from build123d import *

# Parameters (mm, degrees)
BOX011_W          = 6.2
BOX011_H          = 10
BOX011_DEPTH      = 2.4
BOX010_W          = 6.2
BOX010_H          = 10
BOX010_DEPTH      = 2.4
CYLINDER007_R     = 1.5
CYLINDER007_DEPTH = 60
CYLINDER006_R     = 4.5
CYLINDER006_DEPTH = 60


with BuildPart() as nut2:
    # Box011 → Box011 (new body)
    with BuildSketch(Plane(origin=(-3.1, -5, 51.6), x_dir=(1, 0, 0), z_dir=(0, 0, 1))):
        with Locations((3.1, 5)):
            Rectangle(BOX011_W, BOX011_H)
    extrude(amount=BOX011_DEPTH)


with BuildPart() as nut1:
    # Box010 → Box010 (new body)
    with BuildSketch(Plane(origin=(-3.1, -5, 6), x_dir=(1, 0, 0), z_dir=(0, 0, 1))):
        with Locations((3.1, 5)):
            Rectangle(BOX010_W, BOX010_H)
    extrude(amount=BOX010_DEPTH)


with BuildPart() as columnhole:
    # Cylinder007 → Cylinder007 (new body)
    with BuildSketch(Plane.XY):
        Circle(CYLINDER007_R)
    extrude(amount=CYLINDER007_DEPTH)


with BuildPart() as column:
    # Cylinder006 → Cylinder006 (new body)
    with BuildSketch(Plane.XY):
        Circle(CYLINDER006_R)
    extrude(amount=CYLINDER006_DEPTH)

    # Cut010: cut ColumnHole
    add(columnhole.part, mode=Mode.SUBTRACT)

    # Cut011: cut Nut1
    add(nut1.part, mode=Mode.SUBTRACT)

    # Cut012: cut Nut2
    add(nut2.part, mode=Mode.SUBTRACT)


solid = column.part
The listing builds one solid part. Answer for the finished solid, in the listing's coordinates (mm). A direction names the side the tool comes from. Round coordinates to 2 decimals unless told otherwise and drop trailing zeros. Loops run counter-clockwise (first coordinate to the right, second up) from the corner with the lowest first, then second, coordinate; pieces in that order, holes last. Notation, with made-up numbers: M 45.25,-34 L 73.25,-34 A32 cw 73.25,4 Z; hole C 13.25,86.5 d1. An arc over 180 degrees is marked long. Return JSON: item names as keys, results as strings.
Q1. Find the intervals of material crossed by line 1 along Z through (x, y) = (-2, 3); line 2 along Y through (x, z) = (0, 49); line 3 along X through (y, z) = (-0.75, 33), in increasing order. Write a range as from..to.
Results list:
{"line 1": "z = 0..6, 8.4..51.6, 54..60", "line 2": "y = -4.5..-1.5, 1.5..4.5", "line 3": "x = -4.44..-1.3, 1.3..4.44"}
Q2. Find section A-A, the plane x = 0. Determine the outline of the cut face in (y, z), plus the area to 3 significant figures.
Results list:
{"outline": "M -4.5,0 L -1.5,0 L -1.5,6 L -4.5,6 Z; M -4.5,8.4 L -1.5,8.4 L -1.5,51.6 L -4.5,51.6 Z; M -4.5,54 L -1.5,54 L -1.5,60 L -4.5,60 Z; M 1.5,0 L 4.5,0 L 4.5,6 L 1.5,6 Z; M 1.5,8.4 L 4.5,8.4 L 4.5,51.6 L 1.5,51.6 Z; M 1.5,54 L 4.5,54 L 4.5,60 L 1.5,60 Z", "area": "331 mm2"}
Q3. Find section B-B, the plane y = 0.5. Determine the outline of the cut face in (x, z).
Results list:
{"outline": "M -4.47,0 L -1.41,0 L -1.41,6 L -3.1,6 L -3.1,8.4 L -1.41,8.4 L -1.41,51.6 L -3.1,51.6 L -3.1,54 L -1.41,54 L -1.41,60 L -4.47,60 Z; M 1.41,0 L 4.47,0 L 4.47,60 L 1.41,60 L 1.41,54 L 3.1,54 L 3.1,51.6 L 1.41,51.6 L 1.41,8.4 L 3.1,8.4 L 3.1,6 L 1.41,6 Z"}
Q4. Find section C-C, the plane x = 2.5. Determine the outline of the cut face in (y, z).
Results list:
{"outline": "M -3.74,0 L 3.74,0 L 3.74,6 L -3.74,6 Z; M -3.74,8.4 L 3.74,8.4 L 3.74,51.6 L -3.74,51.6 Z; M -3.74,54 L 3.74,54 L 3.74,60 L -3.74,60 Z"}
Q5. Find section D-D, the plane z = 53. Determine the outline of the cut face in (x, y), plus the area to 3 significant figures.
Results list:
{"outline": "M -3.1,-3.26 L -3.1,3.26 A4.5 ccw Z; M 3.1,-3.26 A4.5 ccw 3.1,3.26 Z", "area": "12.6 mm2"}
Q6. The mould has two halves that part along X. Classify faces 3 (the face through (3.1, 0, 53)), 4 (the face through (-1.5, 0.07, 29.7)), 5 (the face through (0, -2, 0)), 6 (the face through (-0.59, 4.46, 29.58)): released by +X, released by -X, zero draft, split by the parting line, or undercut.
Results list:
{"face 3": "undercut", "face 4": "undercut", "face 5": "zero draft", "face 6": "split by the parting line"}
Q7. Each of these flat-tipped pins is pushed along its axis until it touches: pin 1 Ø1.8 at (x, y) = (0, 0) entering from +Z; pin 2 Ø0.7 at (y, z) = (0.5, 52.5) entering from -X; pin 3 Ø1.9 at (y, z) = (1.5, 6.5) entering from +X. Where does it stop, or does it pass through?
Results list:
{"pin 1": "passes through", "pin 2": "stops at x = -4.5", "pin 3": "stops at x = 4.47"}
Q8. Which of the six approach directions +Z, -Z, +X, -X, +Y, -Y give full straight-line access (tool end or side, diameter ignored) to faces 1 (the face through (-1.5, 0.07, 2.96)), 2 (the face through (3.1, 0, 7))?
Results list:
{"face 1": "+Z, -Z", "face 2": "+Y, -Y"}
